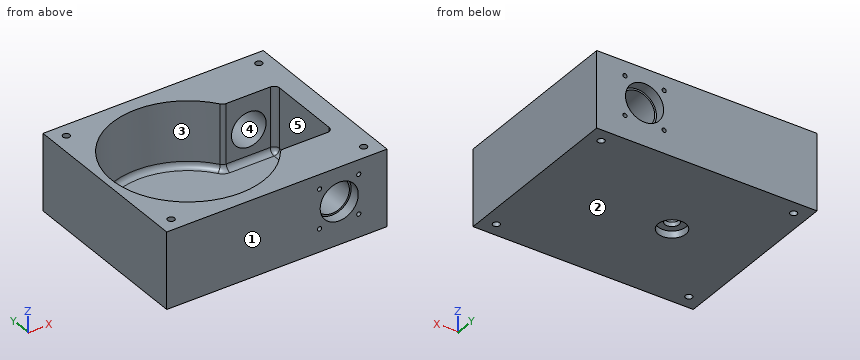
from build123d import *

# Parameters (mm, degrees)
F2_W      = 201.93
F2_H      = 70.01637
F3_DEPTH  = 82.55
F5_DEPTH  = 59.69762
F6_R      = 12.7
F7_DEPTH  = 6.35
F8_R      = 6.477
F9_DEPTH  = 25.4
F10_R     = 15.875
F11_DEPTH = 165.101
F12_R     = 3.175
F13_DEPTH = 70.01737
F15_R     = 1.89865
F16_DEPTH = 12.7
F14_R     = 17.4625
F17_DEPTH = 9.525
F18_R     = 5.08


# Not quite as in the source:
# - a pattern or mirror of a feature is missing from the dataset's text; its kind, count and spacing are read off the source's solid


with BuildPart() as f3:
    # F2 (on Front) → F3 (new body, symmetric)
    with BuildSketch(Plane.XZ):
        with Locations((24.765, -3.893185)):
            Rectangle(F2_W, F2_H)
    extrude(amount=F3_DEPTH, both=True)

    # F4 (on face) → F5 (cut)
    with BuildSketch(Plane.XY.offset(31.115)):
        with BuildLine():
            Line((106.68, 38.1), (58.5441073038, 38.1))
            ThreePointArc((58.5441073038, 38.1), (-69.85, 0), (58.5441073038, -38.1))
            Line((58.5441073038, -38.1), (106.68, -38.1))
            Line((106.68, -38.1), (106.68, 38.1))
        make_face()
    extrude(amount=-F5_DEPTH, mode=Mode.SUBTRACT)

    # F6 (on face) → F7 (cut)
    with BuildSketch(Plane(origin=(0, 0, -38.90137), x_dir=(1, 0, 0), z_dir=(0, 0, -1))):
        Circle(F6_R)
    extrude(amount=-F7_DEPTH, mode=Mode.SUBTRACT)

    # F8 (on face) → F9 (cut)
    with BuildSketch(Plane(origin=(0, 0, -32.55137), x_dir=(1, 0, 0), z_dir=(0, 0, -1))):
        Circle(F8_R)
    extrude(amount=-F9_DEPTH, mode=Mode.SUBTRACT)

    # F10 (on face) → F11 (cut, through all)
    with BuildSketch(Plane(origin=(0, 82.55, 0), x_dir=(-1, 0, 0), z_dir=(0, 1, 0))):
        with Locations((-81.915, 0)):
            Circle(F10_R)
    extrude(amount=-F11_DEPTH, mode=Mode.SUBTRACT)

    # F12 (on face) → F13 (cut, through all)
    with BuildSketch(Plane.XY.offset(31.115)):
        with Locations((-63.5, 69.85)):
            Circle(F12_R)
        with Locations((-63.5, -69.85)):
            Circle(F12_R)
        with Locations((113.03, 69.85)):
            Circle(F12_R)
        with Locations((113.03, -69.85)):
            Circle(F12_R)
    extrude(amount=-F13_DEPTH, mode=Mode.SUBTRACT)

    # F15 (on face) → F16 (cut)
    with BuildSketch(Plane(origin=(0, 82.55, 0), x_dir=(-1, 0, 0), z_dir=(0, 1, 0))):
        with Locations((-99.8755122421, 17.9605122421)):
            Circle(F15_R)
        with Locations((-99.8755122421, -17.9605122421)):
            Circle(F15_R)
        with Locations((-63.9544877579, -17.9605122421)):
            Circle(F15_R)
        with Locations((-63.9544877579, 17.9605122421)):
            Circle(F15_R)
    f16 = extrude(amount=-F16_DEPTH, mode=Mode.SUBTRACT)

    # F16_copies: F16 across plane
    add(f16.mirror(Plane(origin=(0, 0, 0), x_dir=(0, 0, -1), z_dir=(0, -1, 0))), mode=Mode.SUBTRACT)

    # F14 (on face) → F17 (cut)
    with BuildSketch(Plane(origin=(0, 82.55, 0), x_dir=(-1, 0, 0), z_dir=(0, 1, 0))):
        with Locations((-81.915, 0)):
            Circle(F14_R)
    f17 = extrude(amount=-F17_DEPTH, mode=Mode.SUBTRACT)

    # F17_copies: F17 across plane
    add(f17.mirror(Plane(origin=(0, 0, 0), x_dir=(0, 0, -1), z_dir=(0, -1, 0))), mode=Mode.SUBTRACT)

    # F18
    f18_edges = [f3.edges().sort_by_distance(p)[0] for p in [
        (-69.85, 0, -28.58262),
        (82.612054, 38.1, -28.58262),
        (106.68, 0, -28.58262),
        (82.612054, -38.1, -28.58262),
        (58.544107, 38.1, 1.26619),
        (58.544107, -38.1, 1.26619),
        (106.68, 38.1, 1.26619),
        (106.68, -38.1, 1.26619),
    ]]
    fillet(f18_edges, radius=F18_R)


solid = f3.part
The model under review builds one solid part; all positions refer to its coordinate system, in mm. Face numbers are marked on the shaded views. A direction names the side the tool comes from. Coordinates: 2 decimals unless noted, no trailing zeros. Loops run counter-clockwise (first coordinate to the right, second up) from the corner with the lowest first, then second, coordinate; pieces in that order, holes last. Notation, with made-up numbers: M 71,56 L 101,56 A23 ccw 101,75 Z; hole C -13,-34.75 d1. An arc over 180 degrees is marked long. Put each result on its own line as item: value. Start each with the question number.
Q1. Wall thickness on line 1 (Y direction, x = 0, z = 9); line 2 (Y direction, x = -61, z = -25); line 3 (Y direction, x = -63.5, z = 13) (3 decimals): over which ranges is each line inside the solid? List them lowest first.
Q2. The part is to be moulded in two halves that separate along Y. For the marked faces 1, 2 and 3, say which applies: +Y half, -Y half, draft (parallel to the pull), parting line (faces both ways), or undercut.
Q3. Clearance check with flat-ended pins moving along their axes: pin 1 (19 mm diameter, centred on x = 81.915, z = 0, fed in from +Y); pin 2 (1.1 mm diameter, centred on x = 64, z = -17.5, fed in from -Y); pin 3 (5 mm diameter, centred on x = 7, y = 29.5, fed in from +Z); pin 4 (1.1 mm diameter, centred on x = 64.5, z = 18, fed in from +Y). State where each tip first meets the part, or that it passes through.
Q4. Add section C-C (x = 113.03). Write out the cut boundary in (y, z) (3 decimals), and give its area (3 significant figures).
Q5. Add section B-B (y = 0). Write out the cut boundary in (x, z) (3 decimals), and give its area (3 significant figures).
Q6. For the marked faces 4 and 5, list the 3-axis set-ups (+Z, -Z, +X, -X, +Y, -Y) from which the entire face can be reached by the end or side of a thin tool; tool diameter is ignored.
Q7. Add section A-A (z = 0). Count the separate pieces of the cut face and the enclosed holes in it, and give its area (3 significant figures).
Answers:
1. line 1: y = -82.55 to -69.85, 69.85 to 82.55
1. line 2: y = -82.55 to -71.81, -67.89 to -33.56, 33.56 to 67.89, 71.81 to 82.55
1. line 3: y = -82.55 to -73.025, -66.675 to -29.099, 29.099 to 66.675, 73.025 to 82.55
2. face 1: -Y half
2. face 2: draft
2. face 3: undercut
3. pin 1: passes through
3. pin 2: stops at y = -69.85
3. pin 3: stops at z = -28.58
3. pin 4: stops at y = 69.85
4. outline: M -82.55,-38.901 L -73.025,-38.901 L -73.025,31.115 L -82.55,31.115 Z; M -66.675,-38.901 L 66.675,-38.901 L 66.675,31.115 L -66.675,31.115 Z; M 73.025,-38.901 L 82.55,-38.901 L 82.55,31.115 L 73.025,31.115 Z
4. area: 10,700 mm^2
5. outline: M -76.2,-38.901 L -12.7,-38.901 L -12.7,-32.551 L -6.477,-32.551 L -6.477,-28.583 L -64.77,-28.583 A5.08 cw -69.85,-23.503 L -69.85,31.115 L -76.2,31.115 Z; M 6.477,-32.551 L 12.7,-32.551 L 12.7,-38.901 L 125.73,-38.901 L 125.73,31.115 L 106.68,31.115 L 106.68,-23.503 A5.08 cw 101.6,-28.583 L 6.477,-28.583 Z
5. area: 3,400 mm^2
6. face 4: +Y, -Y
6. face 5: +Z
7. separate pieces: 2
7. enclosed holes: 4
7. area: 11,900 mm^2
